```python
from build123d import *

# Parameters (mm, degrees)
PAD_DEPTH       = 15.6
SKETCH001_R     = 4.6
PAD001_DEPTH    = 2.7
SKETCH002_R     = 3.35
POCKET_DEPTH    = 2.7
SKETCH003_R     = 2.5
POCKET001_DEPTH = 15.301
SKETCH004_W     = 4.1
SKETCH004_H     = 15.6
PAD002_DEPTH    = 1.8
PAD003_DEPTH    = 10
SKETCH006_R     = 0.875
POCKET002_DEPTH = 8
SKETCH007_R     = 1
POCKET003_DEPTH = 48.501
FILLET_R        = 2
CHAMFER_SIZE    = 0.5
SKETCH008_W     = 16
SKETCH008_H     = 1.8
PAD004_DEPTH    = 1


with BuildPart() as part:
    # Sketch → Pad (new body)
    with BuildSketch(Plane.XY):
        with BuildLine():
            Line((0, 1.8), (0, 0))
            Line((0, 0), (12.300012, 0))
            ThreePointArc((13.5, -1.200002), (13.148533, -0.351477), (12.300012, 0))
            Line((13.5, -1.200002), (13.5, -17.200002))
            ThreePointArc((13.5, -17.200002), (15.491679, -22.008332), (20.300013, -24))
            Line((20.300013, -24), (27.6, -24))
            ThreePointArc((30.8, -27.2), (29.862742, -24.937258), (27.6, -24))
            Line((30.8, -27.2), (30.8, -44.4))
            Line((30.8, -44.4), (38.6, -44.4))
            Line((38.6, -42.6), (38.6, -44.4))
            Line((32.6, -42.6), (38.6, -42.6))
            Line((32.6, -27.2), (32.6, -42.6))
            ThreePointArc((32.6, -27.2), (31.135534, -23.664466), (27.6, -22.2))
            Line((20.300013, -22.2), (27.6, -22.2))
            ThreePointArc((15.3, -17.200002), (16.764472, -20.735539), (20.300013, -22.2))
            Line((15.3, -1.200002), (15.3, -17.200002))
            ThreePointArc((15.3, -1.200002), (14.421326, 0.921315), (12.300012, 1.8))
            Line((0, 1.8), (12.300012, 1.8))
        make_face()
    extrude(amount=PAD_DEPTH)

    # Sketch001 → Pad001 (new body)
    with BuildSketch(Plane.YZ.offset(15.3)):
        with Locations((-6, 7.8)):
            Circle(SKETCH001_R)
    extrude(amount=PAD001_DEPTH)

    # Sketch002 → Pocket (cut)
    with BuildSketch(Plane.YZ.offset(18)):
        with Locations((-6, 7.8)):
            Circle(SKETCH002_R)
    extrude(amount=-POCKET_DEPTH, mode=Mode.SUBTRACT)

    # Sketch003 → Pocket001 (cut, through all)
    with BuildSketch(Plane.YZ.offset(15.3)):
        with Locations((-6, 7.8)):
            Circle(SKETCH003_R)
    extrude(amount=-POCKET001_DEPTH, mode=Mode.SUBTRACT)

    # Sketch004 → Pad002 (new body)
    with BuildSketch(Plane(origin=(0, 0, 0), x_dir=(0, -1, 0), z_dir=(-1, 0, 0))):
        with Locations((-2.05, 7.8)):
            Rectangle(SKETCH004_W, SKETCH004_H)
    extrude(amount=PAD002_DEPTH)

    # Sketch005 → Pad003 (new body)
    with BuildSketch(Plane.YZ):
        with BuildLine():
            ThreePointArc((1.8, 5.822628), (4.1, 7.8), (1.8, 9.777372))
            Line((1.8, 9.777372), (1.8, 5.822628))
        make_face()
    extrude(amount=PAD003_DEPTH)

    # Sketch006 → Pocket002 (cut)
    with BuildSketch(Plane(origin=(-1.8, 0, 0), x_dir=(0, -1, 0), z_dir=(-1, 0, 0))):
        with Locations((-2, 7.8)):
            Circle(SKETCH006_R)
    extrude(amount=-POCKET002_DEPTH, mode=Mode.SUBTRACT)

    # Sketch007 → Pocket003 (cut, through all)
    with BuildSketch(Plane.XZ.offset(44.4)):
        with Locations((35.6, 11.3)):
            Circle(SKETCH007_R)
        with Locations((35.6, 4.3)):
            Circle(SKETCH007_R)
    extrude(amount=-POCKET003_DEPTH, mode=Mode.SUBTRACT)

    # Fillet
    fillet_edges = [part.edges().sort_by_distance(p)[0] for p in [
        (-0.9, 4.1, 0),
        (-0.9, 4.1, 15.6),
    ]]
    fillet(fillet_edges, radius=FILLET_R)

    # Chamfer
    chamfer_edges = [part.edges().sort_by_distance(p)[0] for p in [
        (18, -9.35, 7.8),
    ]]
    chamfer(chamfer_edges, length=CHAMFER_SIZE)

    # Sketch008 → Pad004 (new body)
    with BuildSketch(Plane(origin=(13.5, 0, 0), x_dir=(0, -1, 0), z_dir=(-1, 0, 0))):
        with Locations((9.200002, 14.7)):
            Rectangle(SKETCH008_W, SKETCH008_H)
        with Locations((9.200002, 0.9)):
            Rectangle(SKETCH008_W, SKETCH008_H)
    extrude(amount=PAD004_DEPTH)


solid = part.part
```
For this review, take the finished solid that the model builds, in its own axes (mm). A direction names the side the tool comes from. Coordinates: 2 decimals unless noted, no trailing zeros. Write each loop counter-clockwise with the first axis right and the second up, starting at its lowest first coordinate (ties: lowest second). Pieces come first, ordered by that corner, then holes.
(1) The part is to be moulded in two halves that separate along Y. For faces 4 (the face through (16.73, -20.7, 7.69)), 5 (the face through (16.42, -6.73, 4.53)), 6 (the face through (24, -24, 8)), 7 (the face through (14.44, 0.9, 7.69)), say which applies: +Y half, -Y half, draft (parallel to the pull), parting line (faces both ways), or undercut.
(2) Add section A-A on y = -6. Give the boundary of the cut face in (x, z), then the cut area to 3 significant figures.
(3) Add section C-C on x = 16.5. Give the boundary of the cut face in (y, z), then the cut area to 3 significant figures.
(4) Tool access review of faces 1 (the face through (15.3, -11, 8)), 2 (the face through (13, -9, 1.8)), 3 (the face through (12.5, -9, 1)): name each direction out of +Z, -Z, +X, -X, +Y, -Y from which nothing blocks a thin tool from reaching the whole face with its end or side.
(5) Add section B-B on x = 35.6. Give the boundary of the cut face in (y, z), then the cut area to 3 significant figures.
(6) Wall thickness on probe 1 along Z at (x, y) = (35.6, -43.35); probe 2 along Z at (x, y) = (14.2, -6); probe 3 along X at (y, z) = (-11, 9.25): over which ranges is each line inside the solid? List them lowest first.
(7) For pin 1 Ø3 at (x, y) = (21, -19) entering from -Z; pin 2 Ø0.9 at (y, z) = (-11, 14.5) entering from -X; pin 3 Ø2.5 at (x, z) = (35.6, 11.3) entering from +Y; pin 4 Ø2.5 at (y, z) = (2.5, 3) entering from +X, all flat-tipped, find the tip position at first contact; note any pin that passes through.
(8) Add section D-D on y = -11.5. Give the boundary of the cut face in (x, z), then the cut area to 3 significant figures.
Answer sheet:
1. face 4: undercut
1. face 5: undercut
1. face 6: -Y half
1. face 7: +Y half
2. outline: (12.5, 0) - (15.3, 0) - (15.3, 3.2) - (18, 3.2) - (18, 3.95) - (17.5, 4.45) - (15.3, 4.45) - (15.3, 5.3) - (13.5, 5.3) - (13.5, 1.8) - (12.5, 1.8) - close; (12.5, 13.8) - (13.5, 13.8) - (13.5, 10.3) - (15.3, 10.3) - (15.3, 11.15) - (17.5, 11.15) - (18, 11.65) - (18, 12.4) - (15.3, 12.4) - (15.3, 15.6) - (12.5, 15.6) - close
2. area: 29.2 mm2
3. outline: (-22.84, 0) - (-20.45, 0) - (-20.45, 15.6) - (-22.84, 15.6) - close; circle Ø9.2 at (-6, 7.8); hole circle Ø6.7 at (-6, 7.8)
3. area: 68.5 mm2
4. face 1: +X
4. face 2: -X, -Y
4. face 3: +Z, -Z, -X, -Y
5. outline: (-44.4, 0) - (-42.6, 0) - (-42.6, 3.3) - (-44.4, 3.3) - close; (-44.4, 5.3) - (-42.6, 5.3) - (-42.6, 10.3) - (-44.4, 10.3) - close; (-44.4, 12.3) - (-42.6, 12.3) - (-42.6, 15.6) - (-44.4, 15.6) - close
5. area: 20.9 mm2
6. probe 1: z = 0 to 3.3, 5.3 to 10.3, 12.3 to 15.6
6. probe 2: z = 0 to 5.3, 10.3 to 15.6
6. probe 3: x = 13.5 to 15.3
7. pin 1: passes through
7. pin 2: stops at x = 12.5
7. pin 3: stops at y = -42.6
7. pin 4: stops at x = 14.03
8. outline: (12.5, 0) - (15.3, 0) - (15.3, 15.6) - (12.5, 15.6) - (12.5, 13.8) - (13.5, 13.8) - (13.5, 1.8) - (12.5, 1.8) - close
8. area: 31.7 mm2
